For this review, use the dimensioned drawing (mm, ordinates from the lowest corner) and the shaded views. A direction names the side the tool comes from. Round coordinates to 2 decimals unless told otherwise and drop trailing zeros. Write each loop counter-clockwise with the first axis right and the second up, starting at its lowest first coordinate (ties: lowest second). Pieces come first, ordered by that corner, then holes. Notation, with made-up numbers: (-24.75, 46) -> (3.25, 46) arc R30 cw to (3.25, 81) -> close; hole circle Ø10 at (66, 59.5). An arc over 180 degrees is marked (long way). Answer as CSV lines item,"result". Start each with the question number.
Item 1: Mouldability with a two-part tool opening along X and no side actions: class the marked faces 1, 2 and 3 as +X half, -X half, draft (parallel to the pull), parting line (faces both ways), or undercut.
Item 2: Take a section at B-B on x = 2.5. Give the boundary of the cut face in (y, z), then the cut area to 4 significant figures.
Item 3: Machinability: for the marked faces 4, 5 and 6, which of the approach directions +Z, -Z, +X, -X, +Y, -Y give a long, thin tool a straight path to every point of the face, cutting with its end or side? Answer none if there is none.
Item 4: For pin 1 Ø2 at (x, y) = (2, 1) entering from -Z; pin 2 Ø2 at (y, z) = (1, 3) entering from -X, all flat-tipped, find the tip position at first contact; note any pin that passes through.
Item 5: Take a section at C-C on y = 2.9. Give the boundary of the cut face in (x, z), then the cut area to 3 significant figures.
Item 6: Take a section at A-A on z = 2.5. Give the boundary of the cut face in (x, y), then the cut area to 4 significant figures.
Item 7: Wall thickness on probe 1 along Z at (x, y) = (2.6, 3.25); probe 2 along Y at (x, z) = (2.05, 2.8); probe 3 along Z at (x, y) = (4.5, 3.4): over which ranges is each line inside the solid? List them lowest first. Write a range as from..to.
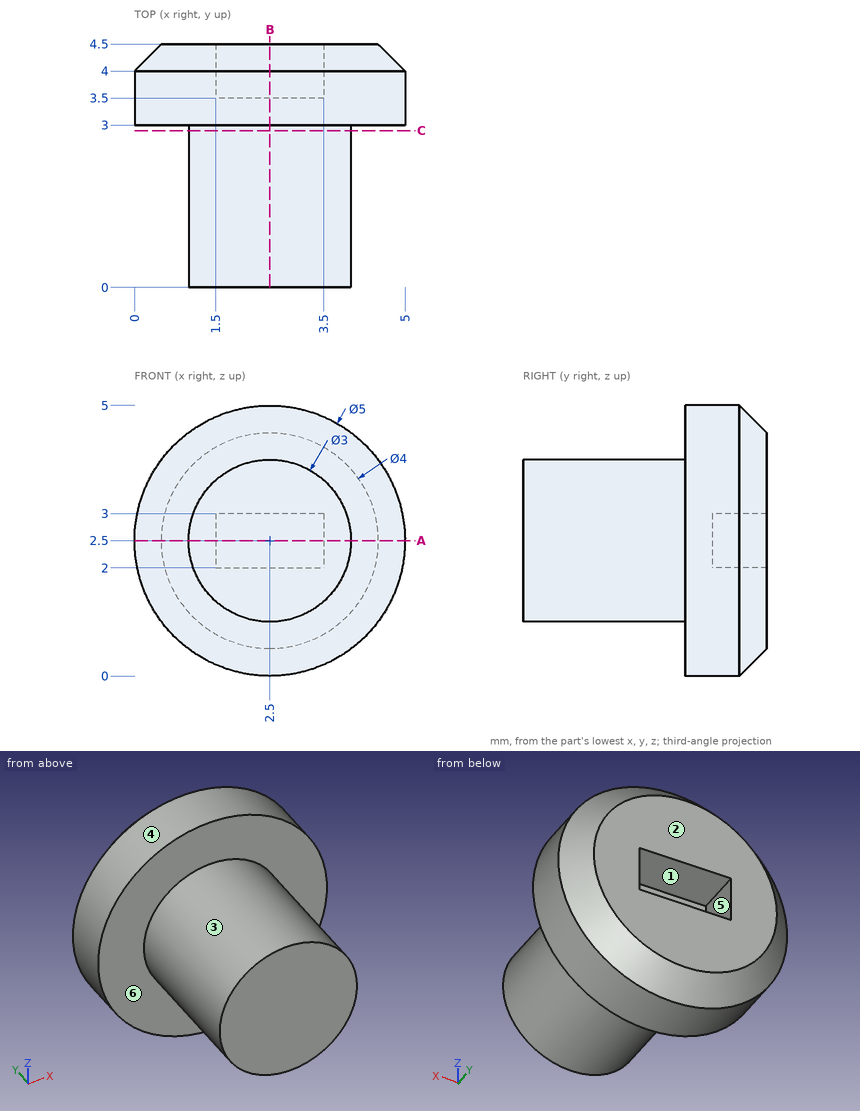
Output values:
1,face 1,"undercut"
1,face 2,"draft"
1,face 3,"parting line"
2,outline,"(0, 1) -> (3, 1) -> (3, 0) -> (4, 0) -> (4.5, 0.5) -> (4.5, 2) -> (3.5, 2) -> (3.5, 3) -> (4.5, 3) -> (4.5, 4.5) -> (4, 5) -> (3, 5) -> (3, 4) -> (0, 4) -> close"
2,area,"15.25 mm^2"
3,face 4,"+Y, -Y"
3,face 5,"+Y"
3,face 6,"-Y"
4,pin 1,"stops at z = 1"
4,pin 2,"stops at x = 1"
5,outline,"circle Ø3 at (2.5, 2.5)"
5,area,"7.07 mm^2"
6,outline,"(0, 3) -> (1, 3) -> (1, 0) -> (4, 0) -> (4, 3) -> (5, 3) -> (5, 4) -> (4.5, 4.5) -> (3.5, 4.5) -> (3.5, 3.5) -> (1.5, 3.5) -> (1.5, 4.5) -> (0.5, 4.5) -> (0, 4) -> close"
6,area,"14.25 mm^2"
7,probe 1,"z = 0..5"
7,probe 2,"y = 0..3.5"
7,probe 3,"z = 1..4"
